```python
from build123d import *

# Parameters (mm, degrees)
SCALE1_SCALE       = 13.1
SKETCH2_W          = 19.177
SKETCH2_H          = 19.177
CUT_EXTRUDE1_DEPTH = 38.1
SKETCH8_R          = 2.667
CUT_EXTRUDE3_DEPTH = 80.739689811
SKETCH9_R          = 6.35
CUT_EXTRUDE4_DEPTH = 19.05


with BuildPart() as part:
    # Sketch1 → Revolve1 (revolve)
    with BuildSketch(Plane.XY):
        with BuildLine():
            Line((0, 0), (28.575, 0))
            ThreePointArc((28.575, 0), (15.980720366, -2.433262928), (3.175, -3.175))
            ThreePointArc((3.175, -3.175), (0.92993597, -2.24506403), (0, 0))
        make_face()
    revolve(axis=Axis((0, 0, 0), (1, 0, 0)))


with BuildPart() as part_1:
    # Scale1: scaled about (0, 0, 0)
    add(part.part.scale(SCALE1_SCALE))

    # Sketch2 → Cut-Extrude1 (cut)
    with BuildSketch(Plane(origin=(0, 41.91, 0), x_dir=(1, 0, 0), z_dir=(0, 1, 0))):
        with Locations((63.5, 0)):
            Rectangle(SKETCH2_W, SKETCH2_H)
    extrude(amount=-CUT_EXTRUDE1_DEPTH, mode=Mode.SUBTRACT)

    # Sketch8 → Cut-Extrude3 (cut, through all)
    with BuildSketch(Plane(origin=(0, 0, 38.1), x_dir=(-1, 0, 0), z_dir=(0, 0, -1))):
        with Locations((-63.5, 25.4)):
            Circle(SKETCH8_R)
    extrude(amount=CUT_EXTRUDE3_DEPTH, mode=Mode.SUBTRACT)

    # Sketch9 → Cut-Extrude4 (cut)
    with BuildSketch(Plane(origin=(0, 0, 38.1), x_dir=(-1, 0, 0), z_dir=(0, 0, -1))):
        with Locations((-63.5, 25.4)):
            Circle(SKETCH9_R)
    cut_extrude4 = extrude(amount=CUT_EXTRUDE4_DEPTH, mode=Mode.SUBTRACT)

    # Mirror1: Cut-Extrude4 across plane
    add(cut_extrude4.mirror(Plane.XY), mode=Mode.SUBTRACT)


solid = part_1.part
```
CAD build for the part. Positions are in the model's coordinates, mm. A direction names the side the tool comes from. Coordinates: 2 decimals unless noted, no trailing zeros. Write each loop counter-clockwise with the first axis right and the second up, starting at its lowest first coordinate (ties: lowest second). Pieces come first, ordered by that corner, then holes. Notation, with made-up numbers: (-16.5, 8.5) -> (41.5, 8.5) arc R24 ccw to (41.5, 22.5) -> close; hole circle Ø3 at (-13, -40). An arc over 180 degrees is marked (long way). Use CSV: the item, a comma, the result in double quotes. Start each with the question number.
Item 1: Wall check: probe 1 along Y at (x, z) = (63.5, 25); probe 2 along Y at (x, z) = (63.5, 15.5); probe 3 along Z at (x, y) = (38.5, -32). Give the ranges that are in metal, low to high.
Item 2: Band-saw the part on A-A, the plane x = 33. Write the cut outline in (y, z), plus the area to 3 significant figures.
Item 3: Tool access for faces 1 (the flat face through (61, 24, -19.05)), 2 (the cylindrical face through (64.88, 19.2, 26.15)), 3 (the flat face through (53.912, 23, 0)): list every direction of +Z, -Z, +X, -X, +Y, -Y with a clear straight run to the whole face (end or side of a thin tool).
Item 4: Drop flat-ended pins along their axis: P1, Ø20.5, axis at x = 63.5, y = 25.4, coming from the +Z side; P2, Ø10, axis at x = 300.5, y = -16, coming from the -Z side; P3, Ø6, axis at x = 63.5, y = 25.4, coming from the +Z side; P4, Ø1, axis at x = 264, y = -26, coming from the -Z side. Give the stop position or say it passes through.
Item 5: Two-plate mould, pull along Z, no slides. Class faces 4 (the cylindrical face through (64.88, 19.2, -26.15)), 5 (the flat face through (73.088, 23, 0)), 6 (the flat face through (61, 24, 19.05)): +Z half, -Z half, draft (parallel to the pull), parting line (faces both ways), or undercut.
Response values:
1,probe 1,"y = -33.24 to 19.05, 31.75 to 33.24"
1,probe 2,"y = -38.6 to 22.73, 28.07 to 38.6"
1,probe 3,"z = -26.39 to 26.39"
2,outline,"circle Ø81.39 at (0, 0)"
2,area,"5,200 mm2"
3,face 1,"-Z"
3,face 2,"+Z"
3,face 3,"+Y"
4,P1,"stops at z = 38.74"
4,P2,"stops at z = -13.27"
4,P3,"stops at z = 19.05"
4,P4,"passes through"
5,face 4,"draft"
5,face 5,"undercut"
5,face 6,"+Z half"
